Geometry check sheet. Reference: the model listing, model coordinates, mm. Give positions to 0.01 mm unless a question says otherwise; leave off trailing zeros. Write each loop counter-clockwise with the first axis right and the second up, starting at its lowest first coordinate (ties: lowest second). Pieces come first, ordered by that corner, then holes. Notation, with made-up numbers: (10, 77.25) -> (25, 77.25) arc R18 cw to (25, 98.25) -> close; hole circle Ø4 at (82, 40.5). An arc over 180 degrees is marked (long way). Write item = value, one per line. Start each with the question number.
1. Cross-section at B-B, the plane z = 1.35. Record the cut outline in (x, y).
2. Cross-section at D-D, the plane y = -8. Record the cut outline in (x, z), plus the area to 3 significant figures.
3. Thickness scan on line 1 along X through (y, z) = (0.25, 2.6); line 2 along Y through (x, z) = (30, 2.45); line 3 along X through (y, z) = (-1, 2.85). Record the ranges inside material, lowest first.
4. Cross-section at A-A, the plane y = 0. Record the cut outline in (x, z).
5. Cross-section at C-C, the plane x = 27. Record the cut outline in (y, z), plus the area to 3 significant figures.
6. Depth check by flat-ended pin: P1, Ø1, axis at y = 3.5, z = 0.5, coming from the -X side. Enter the tip coordinate at first touch or a pass-through.
7. Mould release check, pull along X, two halves, no side actions. Record for faces 1 (the flat face through (15, 0, 0)), 2 (the cylindrical face through (40, 0, 1)), 3 (the cylindrical face through (3.905, -0.867, 1.521)): pulls with the +X half, pulls with the -X half, needs draft (parallel to the pull), parting line crosses it, or undercut.
Autodesk Inventor part; units mm, degrees
ref_plane "YZ Plane" through (0, 0, 0) normal (1, 0, 0) x (0, 1, 0)
ref_plane "XZ Plane" through (0, 0, 0) normal (0, 1, 0) x (-1, 0, 0)
ref_plane "XY Plane" through (0, 0, 0) normal (0, 0, 1) x (1, 0, 0)
sketch "Szkic1" plane through (0, 0, 0) normal (0, 0, 1) x (1, 0, 0)
  line L0 (0, 0) -> (30, 0) construction
  line L1 (0, -10) -> (30, -10)
  line L2 (30, 10) -> (0, 10)
  arc A0 (0, 10) -> (0, -10) centre (0, 0) ccw
  arc A1 (30, -10) -> (30, 10) centre (30, 0) ccw
  point P0 (15, 0)
  dimension "d0" = 30
  dimension "d1" = 20
extrude "Wyciągnięcie proste1" add sketch "Szkic1" along normal blind 3
hole "Otwór1" at (0, 0, 0) at (30, 0, 0) direction (0, 0, 1) diameter 8 end through all
properties part number "ramie_2_wahacza_tylnego"
Answers:
q1.outline = (0, -10) -> (30, -10) arc R10 ccw to (30, 10) -> (0, 10) arc R10 ccw to start; hole circle Ø8 at (0, 0); hole circle Ø8 at (30, 0)
q2.outline = (-6, 0) -> (36, 0) -> (36, 3) -> (-6, 3) -> close
q2.area = 126 mm^2
q3.line_1 = -10 to -3.99, 3.99 to 26.01, 33.99 to 40
q3.line_2 = -10 to -4, 4 to 10
q3.line_3 = -9.95 to -3.87, 3.87 to 26.13, 33.87 to 39.95
q4.outline = (-10, 0) -> (-4, 0) -> (-4, 3) -> (-10, 3) -> close; (4, 0) -> (26, 0) -> (26, 3) -> (4, 3) -> close; (34, 0) -> (40, 0) -> (40, 3) -> (34, 3) -> close
q5.outline = (-10, 0) -> (-2.65, 0) -> (-2.65, 3) -> (-10, 3) -> close; (2.65, 0) -> (10, 0) -> (10, 3) -> (2.65, 3) -> close
q5.area = 44.1 mm^2
q6.P1 = -9.54
q7.face_1 = needs draft
q7.face_2 = pulls with the +X half
q7.face_3 = undercut
